Job drawing, mm, ordinate dimensions from the low corner. One solid piece. Give positions to 0.01 mm unless a question says otherwise; leave off trailing zeros. Write each loop counter-clockwise with the first axis right and the second up, starting at its lowest first coordinate (ties: lowest second). Pieces come first, ordered by that corner, then holes. Notation, with made-up numbers: (1, 36) -> (29, 36) arc R17 ccw to (29, 42) -> close; hole circle Ø7 at (-39.5, -35). An arc over 180 degrees is marked (long way). Put each result on its own line as item: value. Start each with the question number.
Item 1: Drill centre lines: line 1 along Z through (x, y) = (0.75, 5); line 2 along Z through (x, y) = (5, 6); line 3 along X through (y, z) = (11.75, 0.5). Where is each one in solid material? Low to high.
Item 2: Slice it at C-C, the plane z = 4.5. List the corners of the cut face in (x, y), plus the area to 3 significant figures.
Item 3: Slice it at B-B, the plane x = 0.5. List the corners of the cut face in (y, z), plus the area to 3 significant figures.
Item 4: Flat gauge pins, fed straight in: pin 1 Ø2 at (x, y) = (2.5, 8) entering from -Z; pin 2 Ø0.8 at (x, y) = (7.5, 6) entering from +Z; pin 3 Ø1 at (x, y) = (2.5, 4.5) entering from +Z. Where does each tip first touch, or does it go through?
Item 5: Slice it at A-A, the plane y = 12.25. List the corners of the cut face in (x, z).
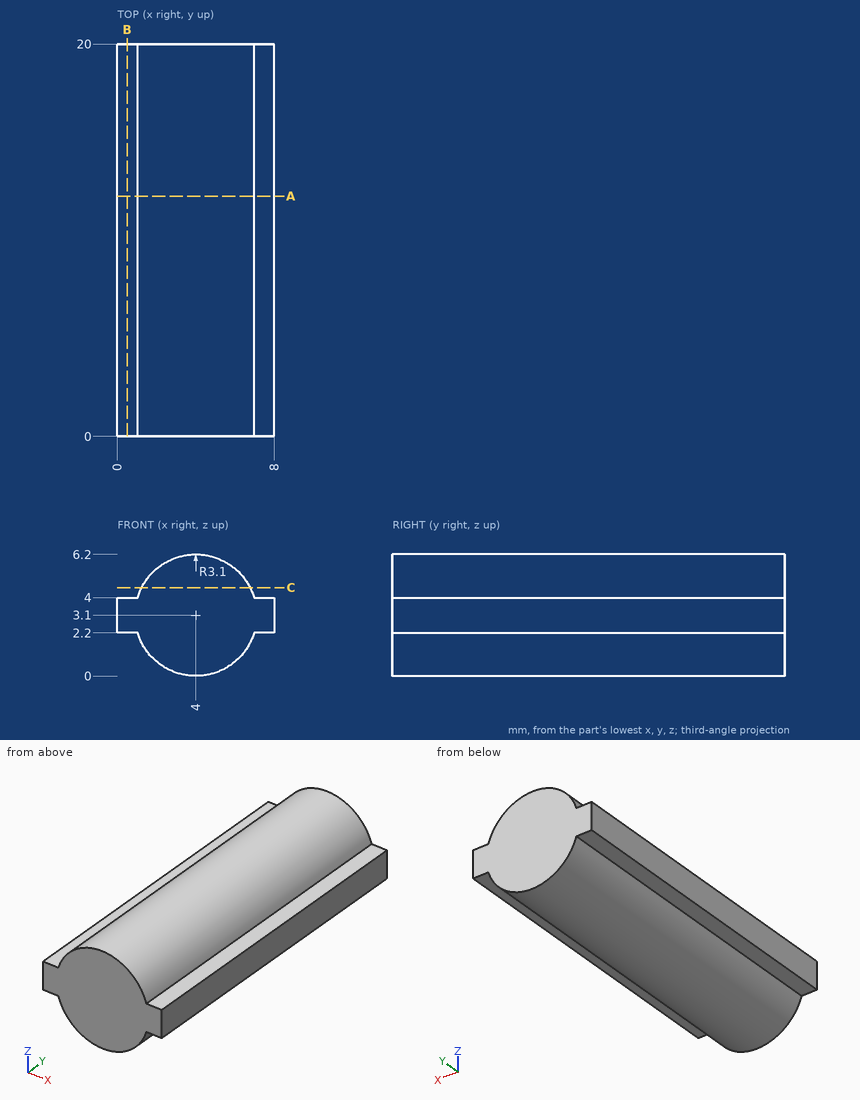
Values follow:
1. line 1: 2.2 to 4
1. line 2: 0.17 to 6.03
1. line 3: 2.31 to 5.69
2. outline: (1.23, 0) -> (6.77, 0) -> (6.77, 20) -> (1.23, 20) -> close
2. area: 111 mm2
3. outline: (0, 2.2) -> (20, 2.2) -> (20, 4) -> (0, 4) -> close
3. area: 36.0 mm2
4. pin 1: z = 0.04
4. pin 2: z = 4
4. pin 3: z = 6.03
5. outline: (0, 2.2) -> (1.03, 2.2) arc R3.1 ccw to (6.97, 2.2) -> (8, 2.2) -> (8, 4) -> (6.97, 4) arc R3.1 ccw to (1.03, 4) -> (0, 4) -> close
